Source: CAD feature listing. Evaluate the final solid. Frame: model axes, mm. A direction names the side the tool comes from. Give positions to 0.01 mm unless a question says otherwise; leave off trailing zeros. Write each loop counter-clockwise with the first axis right and the second up, starting at its lowest first coordinate (ties: lowest second). Pieces come first, ordered by that corner, then holes. Notation, with made-up numbers: (29.25, -28) -> (42.25, -28) arc R21 cw to (42.25, 0) -> close; hole circle Ø5 at (49, -16.5). An arc over 180 degrees is marked (long way). Write item = value, one per line.
from build123d import *

# Parameters (mm, degrees)
F1_DEPTH = 76.2
F3_DEPTH = 50.8
F4_DEPTH = 76.2
F6_DEPTH = 12.7


with BuildPart() as f1:
    # F0 (on Front) → F1 (new body)
    with BuildSketch(Plane.XZ):
        Polygon((-72.527050972, 12.6634538174), (-72.2392499447, 0), (-33.3512052894, 0), (-33.3512052894, 22.1610423177), (43.4929318726, 22.1610423177), (43.4929318726, 0), (80.2978053689, 0), (80.2978053689, 12.6634538174), (55.8343157172, 12.6634538174), (55.8343157172, 51.2294247746), (-45.1855063438, 51.2294247746), (-45.1855063438, 12.6634538174), align=None)
    extrude(amount=-F1_DEPTH)

    # F2 (on Right) → F3 (cut)
    with BuildSketch(Plane.YZ):
        Polygon((51.5903218925, 51.8050380051), (38.8903218925, 51.8050380051), (26.1903218925, 51.8050380051), (38.8903218925, 42.0196428895), align=None)
    extrude(amount=-F3_DEPTH, mode=Mode.SUBTRACT)

    # F4 (cut): a face of the model
    f4_faces = [f1.faces().sort_by_distance(p)[0] for p in [
        (0, 38.8903218925, 48.1594974796),
    ]]
    extrude(f4_faces, amount=-F4_DEPTH, mode=Mode.SUBTRACT)

    # F5 (on Top) → F6 (cut)
    with BuildSketch(Plane.XY):
        Polygon((55.6040368974, 27.3620393127), (80.5960595608, 0), (80.5960595608, 76.2594789267), (55.6040368974, 50.9958043694), align=None)
    extrude(amount=F6_DEPTH, mode=Mode.SUBTRACT)


solid = f1.part
1) Draft query along Y for faces 6 (the flat face through (-33.351, 38, 11)), 7 (the flat face through (20, 76.2, 32)), 8 (the flat face through (6.03, 44.78, 46.56)), 9 (the flat face through (67.78, 14.03, 6.26)). Return one class per face: pulls with the +Y half, pulls with the -Y half, needs draft (parallel to the pull), parting line crosses it, or undercut.
Computed:
face_6 = needs draft
face_7 = pulls with the +Y half
face_8 = undercut
face_9 = undercut
2) Cut plane A-A (x = 63). Return the cut outline in (y, z), then the cut area to 3 significant figures.
Computed:
outline = (0, 0) -> (19.26, 0) -> (19.26, 12.66) -> (0, 12.66) -> close; (58.47, 0) -> (76.2, 0) -> (76.2, 12.66) -> (58.47, 12.66) -> close
area = 468 mm²
3) Cut plane C-C (y = 8). Return the cut outline in (x, z).
Computed:
outline = (-72.53, 12.66) -> (-72.24, 0) -> (-33.35, 0) -> (-33.35, 22.16) -> (43.49, 22.16) -> (43.49, 0) -> (73.29, 0) -> (73.29, 12.66) -> (55.83, 12.66) -> (55.83, 51.23) -> (-45.19, 51.23) -> (-45.19, 12.66) -> close
4) Access query for faces 1 (the flat face through (6.03, 32.83, 46.69)), 2 (the flat face through (5, 38, 22.161)), 3 (the flat face through (55.604, 39, 6)), 4 (the flat face through (63, 69, 12.663)), 5 (the flat face through (-45.186, 38, 32)). Directions: +Z, -Z, +X, -X, +Y, -Y. A direction counts if a zero-diameter tool reaches every point of the face in a straight line with its end or side. Return the directions, or none.
Computed:
face_1 = +Z, +X, -X
face_2 = -Z, +Y, -Y
face_3 = -Z, +X
face_4 = +Z, +X, +Y, -Y
face_5 = +Z, -X, +Y, -Y
5) Contact query for flat-ended pins moving along their axis: pin 1 (4 mm diameter, centred on y = 21, z = 6, fed in from -X); pin 2 (10 mm diameter, centred on x = -33.5, z = 40, fed in from -Y); pin 3 (19.5 mm diameter, centred on x = 71.5, y = 13, fed in from +Z); pin 4 (1 mm diameter, centred on x = 14, y = 61.5, fed in from -Z). Output: stop coordinate, or through.
Computed:
pin_1 = -72.42
pin_2 = 0
pin_3 = 12.66
pin_4 = 22.16
6) Material intervals for L1, parallel to X at y = 60, z = 18; L2, parallel to X at y = 6.5, z = 37.5; L3, parallel to Z at x = 30.5, y = 17.5, sorted ascending.
Computed:
L1 = -45.19 to -33.35, 43.49 to 55.83
L2 = -45.19 to 55.83
L3 = 22.16 to 51.23
7) Cut plane B-B (x = 11.5). Return the cut outline in (y, z), then the cut area to 3 significant figures.
Computed:
outline = (0, 22.16) -> (76.2, 22.16) -> (76.2, 51.23) -> (50.84, 51.23) -> (38.89, 42.02) -> (26.94, 51.23) -> (0, 51.23) -> close
area = 2,100 mm²
8) Cut plane D-D (z = 31). Return the cut outline in (x, y).
Computed:
outline = (-45.19, 0) -> (55.83, 0) -> (55.83, 76.2) -> (-45.19, 76.2) -> close
